```python
from build123d import *

# Parameters (mm, degrees)
F0_R     = 50.8
F2_R     = 38.1
F4_R     = 6.35
F5_DEPTH = 12.7


with BuildPart() as f3:
    # F0 (on Top) → F3 section 0
    with BuildSketch(Plane.XY):
        Circle(F0_R)
    # F2 (on offset) → F3 section 1
    with BuildSketch(Plane.XY.offset(254)):
        Circle(F2_R)
    loft()

    # F4
    f4_edges = [f3.edges().sort_by_distance(p)[0] for p in [
        (-50.8, 0, 0),
        (44.45, 0, 127),
        (-38.1, 0, 254),
    ]]
    fillet(f4_edges, radius=F4_R)

    # F5 (add): a face of the model
    f5_faces = [f3.faces().sort_by_distance(p)[0] for p in [
        (0, 0, 254),
    ]]
    extrude(f5_faces, amount=F5_DEPTH)


solid = f3.part
```
Source: CAD feature listing. Evaluate the final solid. Frame: model axes, mm. A direction names the side the tool comes from. Give positions to 0.01 mm unless a question says otherwise; leave off trailing zeros. Write each loop counter-clockwise with the first axis right and the second up, starting at its lowest first coordinate (ties: lowest second). Pieces come first, ordered by that corner, then holes.
1. Section query A-A (x = 0). Return the cut outline in (y, z).
2. First-contact query: pin 1 (12 mm diameter, centred on x = 10.5, z = 228, fed in from -Y); pin 2 (10 mm diameter, centred on x = 30, z = 231.5, fed in from -Y); pin 3 (2 mm diameter, centred on y = -14.5, z = 42, fed in from -X). Flat tips, straight axial feed; report the tip coordinate or a pass-through.
3. Material intervals for line 1 along X through (y, z) = (-24, 126); line 2 along X through (y, z) = (30.5, 240); line 3 along Z through (x, y) = (0.5, -33), sorted ascending.
4. Access query for faces 1 (the face through (-6.95, -31.297, 260.261)), 2 (the face through (0, 0, 266.7)). Directions: +Z, -Z, +X, -X, +Y, -Y. A direction counts if a zero-diameter tool reaches every point of the face in a straight line with its end or side. Return the directions, or none.
5. Section query C-C (z = 167.5). Return the cut outline in (x, y) (3 decimals).
6. Section query B-B (z = 209). Return the cut outline in (x, y), then the cut area to 3 significant figures.
Output values:
1. outline: (-50.47, 6.67) arc R6.35 ccw to (-44.12, 0) - (44.12, 0) arc R6.35 ccw to (50.47, 6.67) - (38.4, 247.97) arc R6.35 ccw to (32.06, 254) - (32.06, 266.7) - (-32.06, 266.7) - (-32.06, 254) arc R6.35 ccw to (-38.4, 247.97) - close
2. pin 1: stops at y = -39.2
2. pin 2: stops at y = -30.24
2. pin 3: stops at x = -46.8
3. line 1: x = -37.47 to 37.47
3. line 2: x = -23.98 to 23.98
3. line 3: z = 0 to 253.93
4. face 1: +Z
4. face 2: +Z, +X, -X, +Y, -Y
5. outline: circle Ø84.85 at (0, 0)
6. outline: circle Ø80.7 at (0, 0)
6. area: 5,110 mm2
